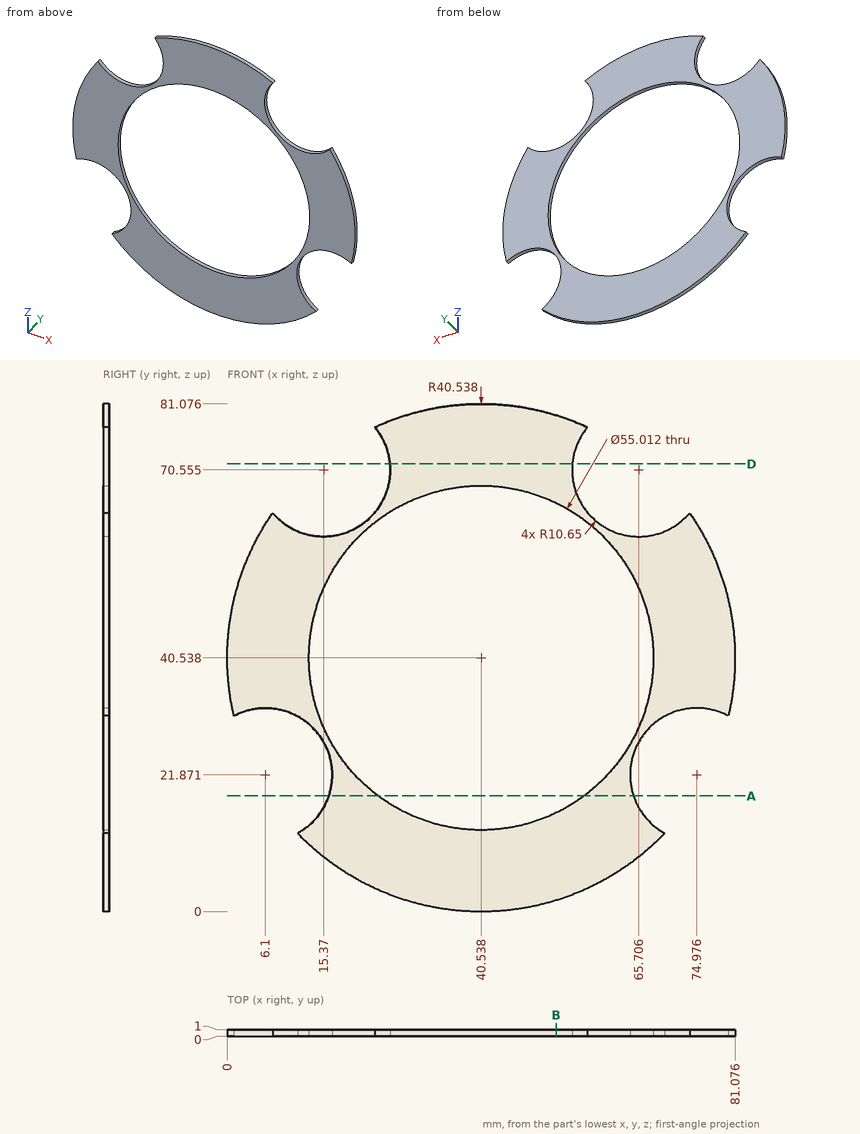
Can you work these out from the drawing? Everything is in mm from the part's minimum corner. Give positions to 0.01 mm unless a question says otherwise; leave off trailing zeros. Loops run counter-clockwise (first coordinate to the right, second up) from the corner with the lowest first, then second, coordinate; pieces in that order, holes last. Notation, with made-up numbers: (-14, 31.5) -> (24, 31.5) arc R18 cw to (24, 60.5) -> close; hole circle Ø4 at (-10, 46.25). An arc over 180 degrees is marked (long way). Return JSON: item names as keys, results as strings.
Item 1: I need wall thicknesses on L1, parallel to X at y = 0.4, z = 41; L2, parallel to Z at x = 25, y = 0.5 (1 decimal); L3, parallel to Z at x = 60.5, y = 0.4 (1 decimal). Which ranges of each line are inside material? Lowest first, please. Write a range as from..to.
Geometry results:
{"L1": "x = 0..13.04, 68.04..81.07", "L2": "z = 3.1..17.8, 63.2..66, 75.1..78", "L3": "z = 5.3..21.6, 59.5..61.3"}
Item 2: If we section it at D-D on z = 71.5: List the corners of the cut face in (x, y) for me.
Geometry results:
{"outline": "(25.98, 0) -> (55.1, 0) -> (55.1, 1) -> (25.98, 1) -> close"}
Item 3: If we section it at B-B on x = 52.5: List the corners of the cut face in (y, z) for me (1 decimal).
Geometry results:
{"outline": "(0, 1.8) -> (1, 1.8) -> (1, 15.8) -> (0, 15.8) -> close; (0, 65.3) -> (1, 65.3) -> (1, 79.3) -> (0, 79.3) -> close"}
Item 4: If we section it at A-A on z = 18.5: List the corners of the cut face in (x, y) for me.
Geometry results:
{"outline": "(16.2, 0) -> (24.08, 0) -> (24.08, 1) -> (16.2, 1) -> close; (57, 0) -> (64.87, 0) -> (64.87, 1) -> (57, 1) -> close"}
